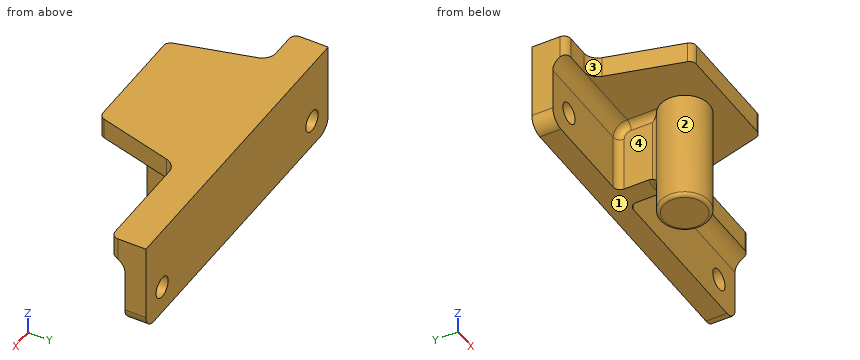
```python
from build123d import *

# Parameters (mm, degrees)
BOSS_EXTRUDE1_DEPTH = 3
SKETCH4_W           = 45
SKETCH4_H           = 3
BOSS_EXTRUDE2_DEPTH = 10
FILLET1_R           = 2
FILLET2_R           = 2
SKETCH5_R           = 1.5
CUT_EXTRUDE1_DEPTH  = 29.702134145
SKETCH6_R           = 3.5
BOSS_EXTRUDE3_DEPTH = 16
FILLET3_R           = 0.5
SKETCH7_W           = 10
SKETCH7_H           = 8.75
BOSS_EXTRUDE4_DEPTH = 1.5
FILLET4_R           = 1


with BuildPart() as part:
    # Sketch3 → Boss-Extrude1 (new body)
    with BuildSketch(Plane.XY):
        with BuildLine():
            Line((2.4, -6), (-12.6, -6))
            ThreePointArc((-12.6, -6), (-13.208761429, -5.79335334), (-13.565925826, -5.258819045))
            Line((-13.565925826, -5.258819045), (-16.386481515, 5.26763809))
            ThreePointArc((-16.386481515, 5.26763809), (-17.100810309, 6.336706681), (-18.318333167, 6.75))
            Line((-18.318333167, 6.75), (-21.5, 6.75))
            ThreePointArc((-21.5, 6.75), (-22.207106781, 7.042893219), (-22.5, 7.75))
            Line((-22.5, 7.75), (-22.5, 11.75))
            Line((-22.5, 11.75), (22.5, 11.75))
            Line((22.5, 11.75), (22.5, 7.75))
            ThreePointArc((22.5, 7.75), (22.207106781, 7.042893219), (21.5, 6.75))
            Line((21.5, 6.75), (8.118333167, 6.75))
            ThreePointArc((8.118333167, 6.75), (6.900810309, 6.336706681), (6.186481515, 5.26763809))
            Line((6.186481515, 5.26763809), (3.365925826, -5.258819045))
            ThreePointArc((3.365925826, -5.258819045), (3.008761429, -5.79335334), (2.4, -6))
        make_face()
    extrude(amount=BOSS_EXTRUDE1_DEPTH)

    # Sketch4 → Boss-Extrude2 (add)
    with BuildSketch(Plane(origin=(0, 0, 0), x_dir=(-1, 0, 0), z_dir=(0, 0, -1))):
        with Locations((0, 10.25)):
            Rectangle(SKETCH4_W, SKETCH4_H)
    extrude(amount=BOSS_EXTRUDE2_DEPTH)

    # Fillet1
    fillet1_edges = [part.edges().sort_by_distance(p)[0] for p in [
        (0, 8.75, 0),
    ]]
    fillet(fillet1_edges, radius=FILLET1_R - 0.0001)  # a hair under: the kernel refuses the full size

    # Fillet2
    fillet2_edges = [part.edges().sort_by_distance(p)[0] for p in [
        (22.5, 10.25, -10),
        (-22.5, 10.25, -10),
    ]]
    fillet(fillet2_edges, radius=FILLET2_R)

    # Sketch5 → Cut-Extrude1 (cut, through all)
    with BuildSketch(Plane.XZ.offset(-8.75)):
        with Locations(Location((-18.5, -6, 0), (0, 0, 270))):
            Circle(SKETCH5_R)
    cut_extrude1 = extrude(amount=-CUT_EXTRUDE1_DEPTH, mode=Mode.SUBTRACT)

    # Mirror1: Cut-Extrude1 across plane
    add(cut_extrude1.mirror(Plane(origin=(0, 0, 0), x_dir=(0, 0, 1), z_dir=(1, 0, 0))), mode=Mode.SUBTRACT)

    # Sketch6 → Boss-Extrude3 (add)
    with BuildSketch(Plane(origin=(0, 0, 0), x_dir=(-1, 0, 0), z_dir=(0, 0, -1))):
        with Locations((5.1, 0)):
            Circle(SKETCH6_R)
    extrude(amount=BOSS_EXTRUDE3_DEPTH)

    # Fillet3
    fillet3_edges = [part.edges().sort_by_distance(p)[0] for p in [
        (-1.6, 0, -16),
    ]]
    fillet(fillet3_edges, radius=FILLET3_R)

    # Sketch7 → Boss-Extrude4 (add, symmetric)
    with BuildSketch(Plane(origin=(-5.1, 0, 0), x_dir=(0, 0, -1), z_dir=(1, 0, 0))):
        with Locations((5, 4.375)):
            Rectangle(SKETCH7_W, SKETCH7_H)
    extrude(amount=BOSS_EXTRUDE4_DEPTH, both=True)

    # Fillet4
    fillet4_edges = [part.edges().sort_by_distance(p)[0] for p in [
        (-3.6, 8.164242852, -0.585757148),
        (-6.6, 4.95618883, 0),
        (-6.6, 8.164242852, -0.585757148),
        (-6.6, 8.75, -5.99995),
        (-3.6, 8.75, -5.99995),
        (-3.6, 4.95618883, 0),
        (-6.6, 3.16227766, -5),
        (-5.1, 3.5, -10),
        (-3.6, 3.16227766, -5),
    ]]
    fillet(fillet4_edges, radius=FILLET4_R)


solid = part.part
```
Read the model definition and answer for the solid it produces. Units are mm, in the model's axes. Face numbers are marked on the shaded views. Coordinates: 2 decimals unless noted, no trailing zeros. Loops run counter-clockwise (first coordinate to the right, second up) from the corner with the lowest first, then second, coordinate; pieces in that order, holes last.
(1) Flat-ended cylindrical pins translate along their axes: pin 1 Ø5 at (x, y) = (5.5, 3) entering from -Z; pin 2 Ø4 at (x, z) = (-18.5, -6) entering from -Y; pin 3 Ø4.5 at (y, z) = (6, -4.5) entering from +X. Find the tip coordinate at first contact, or state that the pin passes through.
Solution:
pin 1: stops at z = 0
pin 2: stops at y = 8.75
pin 3: stops at x = -3.47
(2) The mould has two halves that part along Y. Classify the marked faces 1, 2, 3 and 4: released by +Y, released by -Y, zero draft, split by the parting line, or undercut.
Solution:
face 1: zero draft
face 2: undercut
face 3: released by -Y
face 4: undercut
(3) Consider line 1 along X through (y, z) = (10.1, -6); line 2 along Z through (x, y) = (18.5, 9.4); line 3 along Y through (x, z) = (-7, -7). Determine where each line is inside the solid, lowest interval first.
Solution:
line 1: x = -22.5 to -20, -17 to 17, 20 to 22.5
line 2: z = -10 to -7.5, -4.5 to 3
line 3: y = -2.94 to 2.94, 8.55 to 11.75
(4) The part is cut by section A-A (z = -6). Determine the outline of the cut face in (x, y).
Solution:
outline: (-22.5, 8.75) - (-20, 8.75) - (-20, 11.75) - (-22.5, 11.75) - close; (-17, 8.75) - (-7.6, 8.75) arc R1 cw to (-6.6, 7.75) - (-6.6, 3.74) arc R1 cw to (-7.04, 2.91) arc R3.5 ccw (long way) to (-3.16, 2.91) arc R1 cw to (-3.6, 3.74) - (-3.6, 7.75) arc R1 cw to (-2.6, 8.75) - (17, 8.75) - (17, 11.75) - (-17, 11.75) - close; (20, 8.75) - (22.5, 8.75) - (22.5, 11.75) - (20, 11.75) - close
(5) The part is cut by section D-D (z = -3). Determine the outline of the cut face in (x, y).
Solution:
outline: (-22.5, 8.75) - (-7.6, 8.75) arc R1 cw to (-6.6, 7.75) - (-6.6, 3.74) arc R1 cw to (-7.04, 2.91) arc R3.5 ccw (long way) to (-3.16, 2.91) arc R1 cw to (-3.6, 3.74) - (-3.6, 7.75) arc R1 cw to (-2.6, 8.75) - (22.5, 8.75) - (22.5, 11.75) - (-22.5, 11.75) - close
(6) The part is cut by section C-C (y = 10.5). Determine the outline of the cut face in (x, z).
Solution:
outline: (-22.5, -8) arc R2 ccw to (-20.5, -10) - (20.5, -10) arc R2 ccw to (22.5, -8) - (22.5, 3) - (-22.5, 3) - close; hole circle Ø3 at (-18.5, -6); hole circle Ø3 at (18.5, -6)
